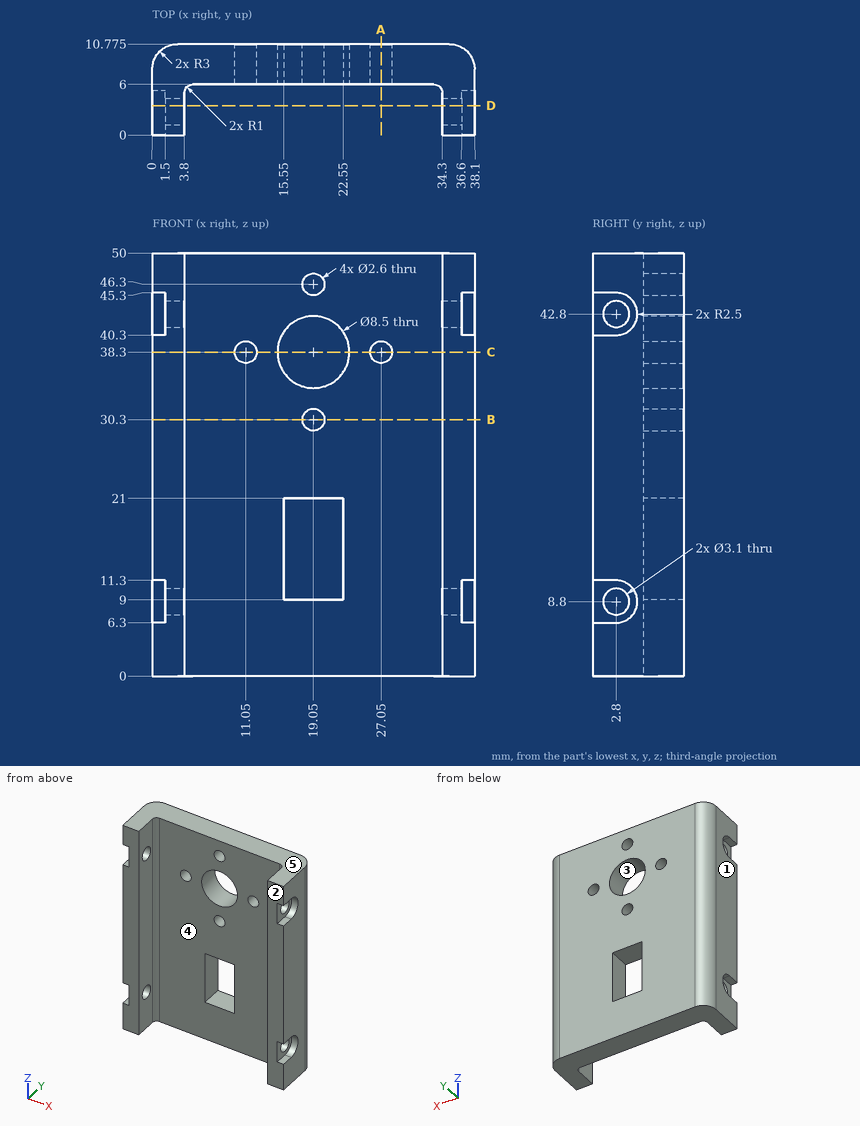
Part print with two shaded views. Sizes in mm from the minimum x, y, z corner. A direction names the side the tool comes from. Give positions to 0.01 mm unless a question says otherwise; leave off trailing zeros. Loops run counter-clockwise (first coordinate to the right, second up) from the corner with the lowest first, then second, coordinate; pieces in that order, holes last. Notation, with made-up numbers: (21.5, -29.5) -> (40.5, -29.5) arc R29 cw to (40.5, -2.5) -> close; hole circle Ø6 at (51.25, 73). An arc over 180 degrees is marked (long way). One line per question, with ' | ' between items.
Q1. Cut at B-B, the plane z = 30.3. Write the cut outline in (x, y) (3 decimals).
Filled sheet:
outline: (0, 0) -> (3.8, 0) -> (3.8, 5) arc R1 cw to (4.8, 6) -> (17.75, 6) -> (17.75, 10.775) -> (3, 10.775) arc R3 ccw to (0, 7.775) -> close; (20.35, 6) -> (33.3, 6) arc R1 cw to (34.3, 5) -> (34.3, 0) -> (38.1, 0) -> (38.1, 7.775) arc R3 ccw to (35.1, 10.775) -> (20.35, 10.775) -> close
Q2. Drill centre lines: line 1 along X through (y, z) = (8.75, 38.3); line 2 along X through (y, z) = (2.25, 30.5); line 3 along X through (y, z) = (7.95, 30.3). Where is each one in solid material? Low to high. Write a range as [from, to].
Filled sheet:
line 1: x = [0.16, 9.75], [12.35, 14.8], [23.3, 25.75], [28.35, 37.94] | line 2: x = [0, 3.8], [34.3, 38.1] | line 3: x = [0.01, 17.75], [20.35, 38.09]
Q3. Pull direction X, two halves, no side cores. Call the marked faces 1, 2 and 3: pulls with the +X half, pulls with the -X half, needs draft (parallel to the pull), parting line crosses it, or undercut.
Filled sheet:
face 1: pulls with the -X half | face 2: needs draft | face 3: undercut
Q4. Cut at A-A, the plane x = 27.05. Write the cut outline in (y, z) (3 decimals).
Filled sheet:
outline: (6, 0) -> (10.775, 0) -> (10.775, 37) -> (6, 37) -> close; (6, 39.6) -> (10.775, 39.6) -> (10.775, 50) -> (6, 50) -> close
Q5. Cut at C-C, the plane z = 38.3. Write the cut outline in (x, y) (3 decimals).
Filled sheet:
outline: (0, 0) -> (3.8, 0) -> (3.8, 5) arc R1 cw to (4.8, 6) -> (9.75, 6) -> (9.75, 10.775) -> (3, 10.775) arc R3 ccw to (0, 7.775) -> close; (12.35, 6) -> (14.8, 6) -> (14.8, 10.775) -> (12.35, 10.775) -> close; (23.3, 6) -> (25.75, 6) -> (25.75, 10.775) -> (23.3, 10.775) -> close; (28.35, 6) -> (33.3, 6) arc R1 cw to (34.3, 5) -> (34.3, 0) -> (38.1, 0) -> (38.1, 7.775) arc R3 ccw to (35.1, 10.775) -> (28.35, 10.775) -> close
Q6. Tool access for the marked faces 4 and 5: list every direction of +Z, -Z, +X, -X, +Y, -Y with a clear straight run to the whole face (end or side of a thin tool).
Filled sheet:
face 4: +Z, -Z, -Y | face 5: +Z, +X, -X, +Y, -Y
Q7. Cut at D-D, the plane y = 3.5. Count the separate pieces of the cut face and the enclosed holes in it, plus the area to 3 significant figures.
Filled sheet:
separate pieces: 6 | enclosed holes: 0 | area: 326 mm²
Q8. Drop flat-ended pins along their axis: pin 1 (1.2 mm diameter, centred on x = 37.5, y = 1.5, fed in from -Z); pin 2 (10 mm diameter, centred on x = 9, z = 44, fed in from -Y); pin 3 (4 mm diameter, centred on y = 2.8, z = 8.8, fed in from -X); pin 4 (5 mm diameter, centred on x = 26, z = 29.5, fed in from -Y). Give the stop position or say it passes through.
Filled sheet:
pin 1: stops at z = 0 | pin 2: stops at y = 5.6 | pin 3: stops at x = 1.5 | pin 4: stops at y = 6
